Check sheet for the modelled part. Datum: model origin and axes. Units: mm. A direction names the side the tool comes from. Round coordinates to 2 decimals unless told otherwise and drop trailing zeros. Order: outer loops, then holes, each group sorted by start corner. A loop starts at its lowest first (then second) coordinate and runs counter-clockwise, first axis right, second up.
from build123d import *

# Parameters (mm, degrees)
EXTRUDE_1_DEPTH     = 75
SKETCH_2_R          = 13
CUT_EXTRUDE_1_DEPTH = 46
SKETCH_3_R          = 11.1
CUT_EXTRUDE_2_DEPTH = 63


with BuildPart() as part:
    # 草图1 → 凸台-拉伸1 (new body)
    with BuildSketch(Plane.XY):
        Polygon((-23.671361037, 0), (-11.835680518, -20.5), (11.835680518, -20.5), (23.671361037, 0), (11.835680518, 20.5), (-11.835680518, 20.5), align=None)
    extrude(amount=EXTRUDE_1_DEPTH)

    # 草图2 → 切除-拉伸1 (cut)
    with BuildSketch(Plane.XY.offset(75)):
        Circle(SKETCH_2_R)
    extrude(amount=-CUT_EXTRUDE_1_DEPTH, mode=Mode.SUBTRACT)

    # 草图3 → 切除-拉伸2 (cut)
    with BuildSketch(Plane.XY.offset(29)):
        Circle(SKETCH_3_R)
    extrude(amount=-CUT_EXTRUDE_2_DEPTH, mode=Mode.SUBTRACT)


solid = part.part
1) Set-up check for faces 1 (the face through (10, 6, 29)), 2 (the face through (10, 9, 75)): record each of +Z, -Z, +X, -X, +Y, -Y from which the full face is reachable in a straight line by a thin tool's end or side.
2) Sectioned sample at C-C on y = -7.5. Record the cut outline in (x, z), and give its area (3 significant figures).
3) Sectioned sample at A-A on x = 0. Record the cut outline in (y, z), and give its area (3 significant figures).
4) Draft check along X on faces 3 (the face through (17.671, -10.394, 36.975)), 4 (the face through (5.97, 9.36, 14.7)), 5 (the face through (0, -20.5, 37)). Enter one of: pulls with the +X half, pulls with the -X half, needs draft (parallel to the pull), parting line crosses it, or undercut.
5) Gauge pin test, flat ends, axial feed: pin 1 (5 mm diameter, centred on y = 7.5, z = 44, fed in from -X); pin 2 (12 mm diameter, centred on x = 1, y = 1, fed in from +Z); pin 3 (5 mm diameter, centred on y = 6, z = 54.5, fed in from -X). Record the tip position at first contact, or that the pin passes through.
6) Sectioned sample at B-B on z = 8.5. Record the cut outline in (x, y), and give its area (3 significant figures).
7) Sectioned sample at D-D on z = 65. Record the cut outline in (x, y), and give its area (3 significant figures).
8) Scan lines: line 1 (Y direction, x = 0, z = 39); line 2 (Y direction, x = 0, z = 11); line 3 (X direction, y = -5, z = 57). Record each from-to range of solid material in increasing order.
Values found:
1. face 1: +Z
1. face 2: +Z, +X, -X, +Y, -Y
2. outline: (-19.34, 0) - (-8.18, 0) - (-8.18, 29) - (-10.62, 29) - (-10.62, 75) - (-19.34, 75) - close; (8.18, 0) - (19.34, 0) - (19.34, 75) - (10.62, 75) - (10.62, 29) - (8.18, 29) - close
2. area: 1,450 mm2
3. outline: (-20.5, 0) - (-11.1, 0) - (-11.1, 29) - (-13, 29) - (-13, 75) - (-20.5, 75) - close; (11.1, 0) - (20.5, 0) - (20.5, 75) - (13, 75) - (13, 29) - (11.1, 29) - close
3. area: 1,240 mm2
4. face 3: pulls with the +X half
4. face 4: undercut
4. face 5: needs draft
5. pin 1: stops at x = -20.78
5. pin 2: passes through
5. pin 3: stops at x = -21.65
6. outline: (-23.67, 0) - (-11.84, -20.5) - (11.84, -20.5) - (23.67, 0) - (11.84, 20.5) - (-11.84, 20.5) - close; hole circle Ø22.2 at (0, 0)
6. area: 1,070 mm2
7. outline: (-23.67, 0) - (-11.84, -20.5) - (11.84, -20.5) - (23.67, 0) - (11.84, 20.5) - (-11.84, 20.5) - close; hole circle Ø26 at (0, 0)
7. area: 925 mm2
8. line 1: y = -20.5 to -13, 13 to 20.5
8. line 2: y = -20.5 to -11.1, 11.1 to 20.5
8. line 3: x = -20.78 to -12, 12 to 20.78
